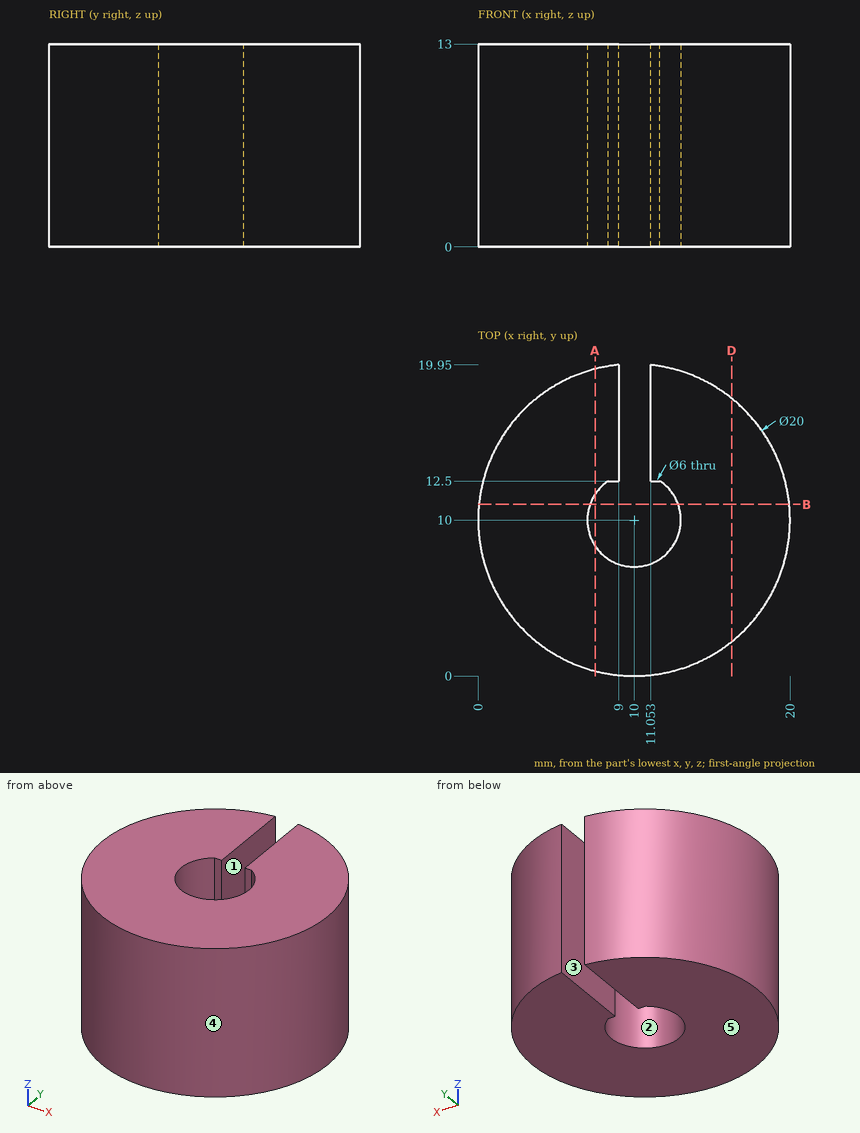
Geometry: see drawing. Coordinates: mm, zero at the bounding-box minimum. A direction names the side the tool comes from. Give positions to 0.01 mm unless a question says otherwise; leave off trailing zeros. Loops run counter-clockwise (first coordinate to the right, second up) from the corner with the lowest first, then second, coordinate; pieces in that order, holes last. Notation, with made-up numbers: (77.5, 8.25) - (127.5, 8.25) arc R22 cw to (127.5, 22.25) - close; hole circle Ø6 at (38.5, 16.25). An arc over 180 degrees is marked (long way). Use CSV: the item, a comma, the result in double quotes.
1) Cut plane B-B (y = 11). Output: boundary loops of the cut face in (x, z), and give its area (3 significant figures).
Worked out:
outline,"(0.05, 0) - (7.17, 0) - (7.17, 13) - (0.05, 13) - close; (12.83, 0) - (19.95, 0) - (19.95, 13) - (12.83, 13) - close"
area,"185 mm^2"
2) Mould query, pull axis X, two halves, no side actions, for the marked faces 3, 4 and 5. Classes: +X half, -X half, draft (parallel to the pull), parting line (faces both ways), or undercut.
Worked out:
face 3,"undercut"
face 4,"parting line"
face 5,"draft"
3) Pin query (flat end, axial travel): P1, Ø3.5, axis at y = 18, z = 7, coming from the -X side (1 decimal); P2, Ø4, axis at x = 15, z = 6, coming from the -Y side; P3, Ø5, axis at y = 15, z = 3.5, coming from the +X side. Return the tip coordinate at first contact, or that it passes through.
Worked out:
P1,"stops at x = 2.2"
P2,"stops at y = 0.46"
P3,"stops at x = 19.68"
4) Line query: line 1 (Y direction, x = 10, z = 2.25); line 2 (X direction, y = 9, z = 2); line 3 (X direction, y = 15.75, z = 7). Output: solid intervals per line, ascending.
Worked out:
line 1,"y = 0 to 7"
line 2,"x = 0.05 to 7.17, 12.83 to 19.95"
line 3,"x = 1.82 to 9, 11.05 to 18.18"
5) Cut plane D-D (x = 16.25). Output: boundary loops of the cut face in (y, z), and give its area (3 significant figures).
Worked out:
outline,"(2.19, 0) - (17.81, 0) - (17.81, 13) - (2.19, 13) - close"
area,"203 mm^2"
6) Set-up query: the marked faces 1 and 2. Return all of +Z, -Z, +X, -X, +Y, -Y with unobstructed straight access to the full face (end or side cutting, diameter ignored); none if empty.
Worked out:
face 1,"+Z, -Z, +Y"
face 2,"+Z, -Z"
7) Cut plane A-A (x = 7.5). Output: boundary loops of the cut face in (y, z), and give its area (3 significant figures).
Worked out:
outline,"(0.32, 0) - (8.34, 0) - (8.34, 13) - (0.32, 13) - close; (11.66, 0) - (19.68, 0) - (19.68, 13) - (11.66, 13) - close"
area,"209 mm^2"
